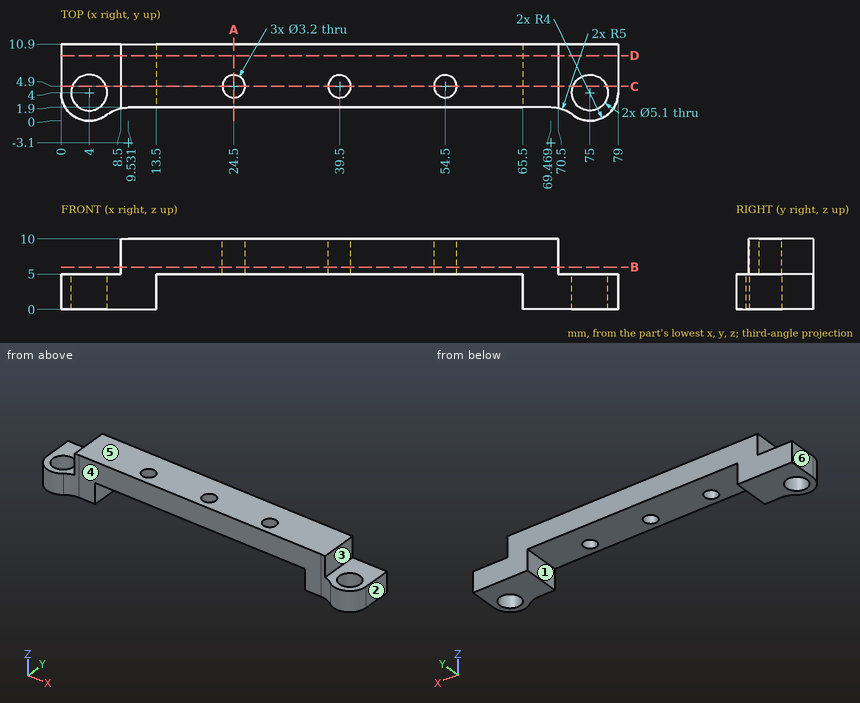
Design review of the part shown in the three views and the two pictorial views. Dimensions are in mm from the part's minimum x, y and z. A direction names the side the tool comes from. Give positions to 0.01 mm unless a question says otherwise; leave off trailing zeros. Loops run counter-clockwise (first coordinate to the right, second up) from the corner with the lowest first, then second, coordinate; pieces in that order, holes last. Notation, with made-up numbers: (30.25, 66.5) - (64.25, 66.5) arc R15 cw to (64.25, 82.5) - close; hole circle Ø3 at (55, 46). An arc over 180 degrees is marked (long way). Answer as a JSON object with one key per item and string values.
Q1. Insertion check: pin 1 (1.5 mm diameter, centred on x = 69, z = 7, fed in from -Y); pin 2 (2.5 mm diameter, centred on y = 5.5, z = 7, fed in from -X); pin 3 (1.5 mm diameter, centred on x = 56, y = 9, fed in from -Z). Each pin has a flat end and moves straight along its axis. Give the tip position at first contact, or say it passes through.
Worked out:
{"pin 1": "stops at y = 1.89", "pin 2": "stops at x = 8.5", "pin 3": "stops at z = 5"}
Q2. To check wall thickness, follow line 1 along Y through (x, z) = (4, 2.8); line 2 along Y through (x, z) = (24.5, 8.35); line 3 along X through (y, z) = (10.5, 1). State the ranges of each line that lie inside material, in increasing order.
Worked out:
{"line 1": "y = 0 to 1.45, 6.55 to 10.9", "line 2": "y = 1.9 to 3.3, 6.5 to 10.9", "line 3": "x = 0 to 13.5, 65.5 to 79"}
Q3. Mouldability with a two-part tool opening along X and no side actions: class the marked faces 4, 5 and 6 as +X half, -X half, draft (parallel to the pull), parting line (faces both ways), or undercut.
Worked out:
{"face 4": "undercut", "face 5": "draft", "face 6": "-X half"}
Q4. Add section A-A on x = 24.5. State the section outline as (y, z) points.
Worked out:
{"outline": "(1.9, 5) - (3.3, 5) - (3.3, 10) - (1.9, 10) - close; (6.5, 5) - (10.9, 5) - (10.9, 10) - (6.5, 10) - close"}
Q5. For the marked faces 1, 2 and 3, list the 3-axis set-ups (+Z, -Z, +X, -X, +Y, -Y) from which the entire face can be reached by the end or side of a thin tool; tool diameter is ignored.
Worked out:
{"face 1": "-Z, +Y, -Y", "face 2": "+Z, -Z, +X, +Y, -Y", "face 3": "+Z, +X, +Y, -Y"}
Q6. Add section C-C on y = 4.9. Count the separate pieces of the cut face and the enclosed holes in it, plus the area to 3 significant figures.
Worked out:
{"separate pieces": "6", "enclosed holes": "0", "area": "349 mm^2"}
Q7. Add section D-D on y = 9.25. State the section outline as (x, z) points, plus the area to 3 significant figures.
Worked out:
{"outline": "(0, 0) - (13.5, 0) - (13.5, 5) - (65.5, 5) - (65.5, 0) - (79, 0) - (79, 5) - (70.5, 5) - (70.5, 10) - (8.5, 10) - (8.5, 5) - (0, 5) - close", "area": "445 mm^2"}
Q8. Add section B-B on z = 6. State the section outline as (x, y) points, plus the area to 3 significant figures.
Worked out:
{"outline": "(8.5, 1.79) arc R5 cw to (9.53, 1.9) - (69.47, 1.9) arc R5 cw to (70.5, 1.79) - (70.5, 10.9) - (8.5, 10.9) - close; hole circle Ø3.2 at (24.5, 4.9); hole circle Ø3.2 at (39.5, 4.9); hole circle Ø3.2 at (54.5, 4.9)", "area": "534 mm^2"}
